Geometry: see drawing. Coordinates: mm, zero at the bounding-box minimum. A direction names the side the tool comes from. Coordinates: 2 decimals unless noted, no trailing zeros. Order: outer loops, then holes, each group sorted by start corner. A loop starts at its lowest first (then second) coordinate and runs counter-clockwise, first axis right, second up. Notation, with made-up numbers: (-9.75, -2.75) -> (45.25, -2.75) arc R16 cw to (45.25, 25.25) -> close; hole circle Ø1 at (12.5, 24). An arc over 180 degrees is marked (long way). Use one line per item in the form item = value.
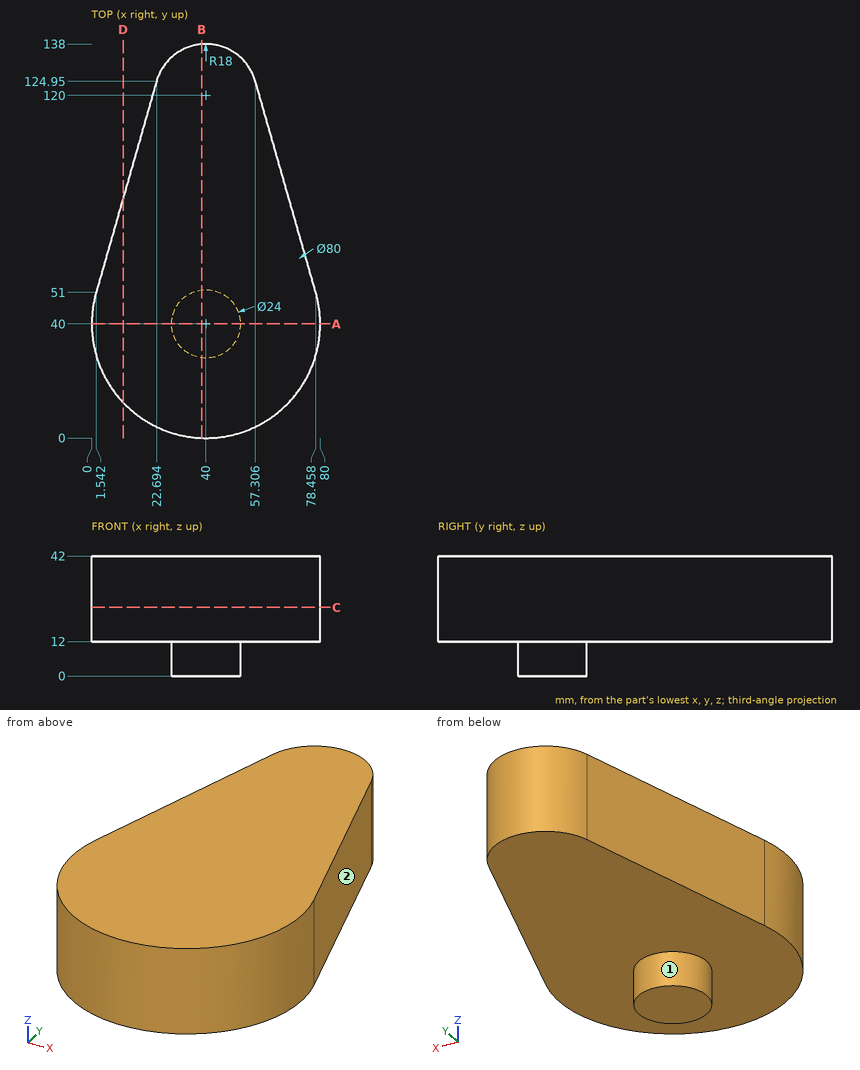
1) Section C-C, the plane z = 24. Output: boundary loops of the cut face in (x, y), and give its area (3 significant figures).
Results found:
outline = (1.54, 51) arc R40 ccw (long way) to (78.46, 51) -> (57.31, 124.95) arc R18 ccw to (22.69, 124.95) -> close
area = 7,840 mm2
2) Material intervals for probe 1 along Z at (x, y) = (25.5, 77.5); probe 2 along X at (y, z) = (108.5, 26); probe 3 along Y at (x, z) = (33.5, 11), sorted ascending. Write a range as from..to.
Results found:
probe_1 = 12..42
probe_2 = 17.99..62.01
probe_3 = 29.91..50.09
3) Contact query for flat-ended pins moving along their axis: P1, Ø3, axis at x = 8.5, y = 51, coming from the -Z side; P2, Ø8, axis at y = 115.5, z = 34.5, coming from the +X side; P3, Ø2, axis at y = 53, z = 14, coming from the +X side. Output: stop coordinate, or through.
Results found:
P1 = 12
P2 = 61.15
P3 = 78.17
4) Section B-B, the plane x = 38.5. Output: boundary loops of the cut face in (y, z), and give its area (3 significant figures).
Results found:
outline = (0.03, 12) -> (28.09, 12) -> (28.09, 0) -> (51.91, 0) -> (51.91, 12) -> (137.94, 12) -> (137.94, 42) -> (0.03, 42) -> close
area = 4,420 mm2
5) Section A-A, the plane y = 40. Output: boundary loops of the cut face in (x, z).
Results found:
outline = (0, 12) -> (28, 12) -> (28, 0) -> (52, 0) -> (52, 12) -> (80, 12) -> (80, 42) -> (0, 42) -> close
6) Access query for the marked faces 1 and 2. Directions: +Z, -Z, +X, -X, +Y, -Y. A direction counts if a zero-diameter tool reaches every point of the face in a straight line with its end or side. Return the directions, or none.
Results found:
face_1 = -Z
face_2 = +Z, -Z, +X, +Y
7) Section D-D, the plane x = 11. Output: boundary loops of the cut face in (y, z).
Results found:
outline = (12.45, 12) -> (84.07, 12) -> (84.07, 42) -> (12.45, 42) -> close
